```python
from build123d import *

# Parameters (mm, degrees)
F1_DEPTH = 63.5
F0_W     = 18.9016429644
F0_H     = 19.05
F0_H_2   = 4.7498
F0_H_3   = 4.7752
F2_DEPTH = 25.4
F3_DEPTH = 7.9375


with BuildPart() as f1:
    # F0 (on Front) → F1 (new body, symmetric)
    with BuildSketch(Plane.XZ):
        Polygon((41.275, -9.525), (41.275, 9.525), (22.225, 9.525), (-41.275, 9.525), (-41.275, -9.525), align=None)
    extrude(amount=F1_DEPTH, both=True)

    # F0 (on Front) → F2 (join, symmetric)
    with BuildSketch(Plane.XZ):
        with BuildLine():
            Line((22.225, 9.525), (41.275, 9.525))
            Line((41.275, 9.525), (41.275, 27.0002))
            ThreePointArc((41.275, 27.0002), (45.9246798487, 38.2255201513), (57.15, 42.8752))
            Line((57.15, 42.8752), (66.8233570356, 42.8752))
            Line((66.8233570356, 42.8752), (66.8233570356, 61.9252))
            Line((66.8233570356, 61.9252), (57.15, 61.9252))
            ThreePointArc((57.15, 61.9252), (32.4542956671, 51.6959043329), (22.225, 27.0002))
            Line((22.225, 27.0002), (22.225, 9.525))
        make_face()
        with Locations((76.2741785178, 52.4002)):
            Rectangle(F0_W, F0_H)
        Polygon((85.725, 61.9252), (85.725, 42.8752), (85.725, 38.1), (104.6266429644, 38.1), (104.6266429644, 66.675), (85.725, 66.675), align=None)
        with Locations((76.2741785178, 64.3001)):
            Rectangle(F0_W, F0_H_2)
        with Locations((76.2741785178, 40.4876)):
            Rectangle(F0_W, F0_H_3)
    extrude(amount=F2_DEPTH, both=True)

    # F0 (on Front) → F3 (join, symmetric)
    with BuildSketch(Plane.XZ):
        with BuildLine():
            Line((-41.275, 9.525), (22.225, 9.525))
            Line((22.225, 9.525), (22.225, 27.0002))
            ThreePointArc((22.225, 27.0002), (32.4542956671, 51.6959043329), (57.15, 61.9252))
            add(Edge.make_bspline(
                [(-41.275, 9.525), (-44.257581234, 40.212534368), (19.0355218947, 67.5760954618), (57.15, 61.9252)],
                knots=[0, 0, 0, 0, 111.5045361635, 111.5045361635, 111.5045361635, 111.5045361635], degree=3))
        make_face()
    extrude(amount=F3_DEPTH, both=True)


solid = f1.part
```
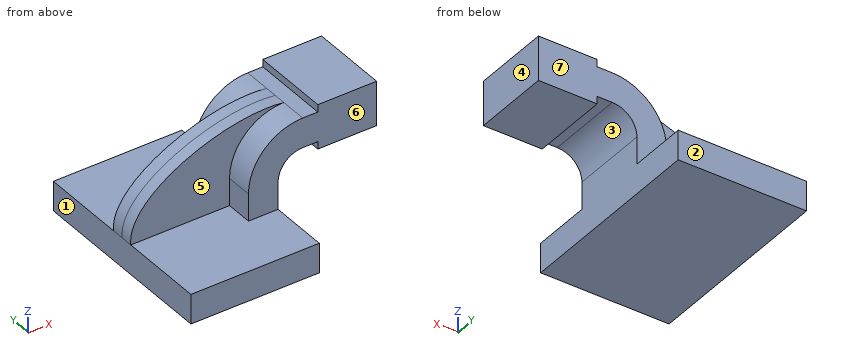
Input: part model. Units: mm. Frame: model coordinates. Face numbers are marked on the shaded views. A direction names the side the tool comes from. Coordinates: 2 decimals unless noted, no trailing zeros. Loops run counter-clockwise (first coordinate to the right, second up) from the corner with the lowest first, then second, coordinate; pieces in that order, holes last. Notation, with made-up numbers: M 8.25,71.25 L 19.25,71.25 A20 cw 19.25,110.25 Z; hole C -9.5,52.5 d8. An arc over 180 degrees is marked long. Use a Markdown table: item, result. Add a question column.
1) Line query: L1, parallel to Z at x = 2, y = -30 (3 decimals); L2, parallel to X at y = 13, z = 27.5; L3, parallel to Y at x = 24, z = 42.5. Output: solid intervals per line, ascending. Write a range as from..to.
2) Set-up query: the marked faces 5, 6 and 7. Return all of +Z, -Z, +X, -X, +Y, -Y with unobstructed straight access to the full face (end or side cutting, diameter ignored); none if empty.
3) Section C-C, the plane x = 95.5. Return the cut outline in (y, z) (3 decimals), plus the area to 3 significant figures.
4) Section A-A, the plane y = 16.5. Return the cut outline in (x, z) (3 decimals).
5) Pin query (flat end, axial travel): P1, Ø19, axis at y = -18.5, z = 20.5, coming from the -X side (3 decimals); P2, Ø2.5, axis at y = -1.5, z = 64.5, coming from the -X side; P3, Ø5.5, axis at y = 7.5, z = 39.5, coming from the -X side; P4, Ø17, axis at x = 54.5, z = 30, coming from the -Y side. Return the tip coordinate at first contact, or that it passes through.
6) Draft query along X for the marked faces 1, 2, 3 and 4. Return one class per face: +X half, -X half, draft (parallel to the pull), parting line (faces both ways), or undercut.
7) Section B-B, the plane z = 7. Return the cut outline in (x, y) (3 decimals), plus the area to 3 significant figures.
Answer below:
| question | item | result |
|---|---|---|
| 1 | L1 | -9.525..9.525 |
| 1 | L2 | 22.23..41.28 |
| 1 | L3 | -7.94..7.94 |
| 2 | face 5 | +Z, -X, -Y |
| 2 | face 6 | +Z, +X, -X, -Y |
| 2 | face 7 | +Z, +X, -X, +Y |
| 3 | outline | M -25.4,38.1 L 25.4,38.1 L 25.4,66.675 L -25.4,66.675 Z |
| 3 | area | 1,450 mm2 |
| 4 | outline | M -41.275,-9.525 L 41.275,-9.525 L 41.275,27 A15.875 cw 57.15,42.875 L 66.823,42.875 L 66.823,38.1 L 104.627,38.1 L 104.627,66.675 L 66.823,66.675 L 66.823,61.925 L 57.15,61.925 A34.925 ccw 22.225,27 L 22.225,9.525 L -41.275,9.525 Z |
| 5 | P1 | x = 22.225 |
| 5 | P2 | x = 66.82 |
| 5 | P3 | x = -27.06 |
| 5 | P4 | through |
| 6 | face 1 | -X half |
| 6 | face 2 | draft |
| 6 | face 3 | undercut |
| 6 | face 4 | +X half |
| 7 | outline | M -41.275,-63.5 L 41.275,-63.5 L 41.275,63.5 L -41.275,63.5 Z |
| 7 | area | 10,500 mm2 |
